The listing builds one solid part. Answer for the finished solid, in the listing's coordinates (mm). A direction names the side the tool comes from. Round coordinates to 2 decimals unless told otherwise and drop trailing zeros. Order: outer loops, then holes, each group sorted by start corner. A loop starts at its lowest first (then second) coordinate and runs counter-clockwise, first axis right, second up. Notation, with made-up numbers: (74, 76) - (96, 76) arc R21 ccw to (96, 90) - close; hole circle Ø6 at (-24.5, 89). An arc over 180 degrees is marked (long way). Write item = value, one per line.
from build123d import *

# Parameters (mm, degrees)
SKETCH1_R           = 11
BOSS_EXTRUDE1_DEPTH = 8
SKETCH2_R           = 11
SKETCH2_R_2         = 2.55
BOSS_EXTRUDE2_DEPTH = 4
CHAMFER1_SIZE       = 1


with BuildPart() as part:
    # Sketch1 → Boss-Extrude1 (new body)
    with BuildSketch(Plane.XY):
        Circle(SKETCH1_R)
        Polygon((4.05, 2.33826859), (0, 4.67653718), (-4.05, 2.33826859), (-4.05, -2.33826859), (0, -4.67653718), (4.05, -2.33826859), align=None, mode=Mode.SUBTRACT)
    extrude(amount=BOSS_EXTRUDE1_DEPTH)

    # Sketch2 → Boss-Extrude2 (add)
    with BuildSketch(Plane.XY.offset(8)):
        Circle(SKETCH2_R)
        Circle(SKETCH2_R_2, mode=Mode.SUBTRACT)
    extrude(amount=BOSS_EXTRUDE2_DEPTH)

    # Chamfer1
    chamfer1_edges = [part.edges().sort_by_distance(p)[0] for p in [
        (-2.025, 3.507402885, 0),
        (-4.05, 0, 0),
        (-2.025, -3.507402885, 0),
        (2.025, -3.507402885, 0),
        (-11, 0, 12),
        (-2.55, 0, 12),
        (4.05, 0, 0),
        (2.025, 3.507402885, 0),
    ]]
    chamfer(chamfer1_edges, length=CHAMFER1_SIZE)


solid = part.part
Q1. Find the intervals of material crossed by line 1 (Y direction, x = 0, z = 9.1); line 2 (X direction, y = 4, z = 4.25); line 3 (Y direction, x = 0.25, z = 2.5), in increasing order. Write a range as from..to.
Model answer:
line_1 = -11..-2.55, 2.55..11
line_2 = -10.25..-1.17, 1.17..10.25
line_3 = -11..-4.53, 4.53..11
Q2. Section B-B on z = 1.75 is taken. Determine the outline of the cut face in (x, y), then the cut area to 3 significant figures.
Model answer:
outline = circle Ø22 at (0, 0); hole (-4.05, -2.34) - (0, -4.68) - (4.05, -2.34) - (4.05, 2.34) - (0, 4.68) - (-4.05, 2.34) - close
area = 323 mm^2
Q3. Section A-A on y = 0 is taken. Determine the outline of the cut face in (x, z), then the cut area to 3 significant figures.
Model answer:
outline = (-11, 0) - (-5.05, 0) - (-4.05, 1) - (-4.05, 8) - (-2.55, 8) - (-2.55, 11) - (-3.55, 12) - (-10, 12) - (-11, 11) - close; (2.55, 8) - (4.05, 8) - (4.05, 1) - (5.05, 0) - (11, 0) - (11, 11) - (10, 12) - (3.55, 12) - (2.55, 11) - close
area = 176 mm^2
Q4. For faces 1 (the face through (2, -5, 0)), 2 (the face through (2, -3.52, 4.45)), determine the directions among +Z, -Z, +X, -X, +Y, -Y from which every point of the face is accessible in a straight line to the end or side of a thin tool.
Model answer:
face_1 = -Z, +X, -X, +Y, -Y
face_2 = -Z
Q5. Determine the mould class of faces 3 (the face through (-2.38, -10.74, 5.42)), 4 (the face through (2, -2, 8)), 5 (the face through (4, 0, 12)), 6 (the face through (1.18, -2.26, 9.48)) for opening direction Y: released by +Y, released by -Y, zero draft, split by the parting line, or undercut.
Model answer:
face_3 = split by the parting line
face_4 = undercut
face_5 = zero draft
face_6 = undercut
Q6. Flat-ended cylindrical pins translate along their axes: P1, Ø3, axis at x = 6, z = 6.5, coming from the -Y side; P2, Ø5, axis at y = 8.5, z = 6, coming from the -X side; P3, Ø1, axis at y = 3.5, z = 3, coming from the +X side; P4, Ø1.4, axis at y = 0.5, z = 3, coming from the +X side. Find the tip coordinate at first contact, or state that the pin passes through.
Model answer:
P1 = -10.04
P2 = -9.22
P3 = 10.58
P4 = 11
